Verification items for the finished model (mm, model axes). A direction names the side the tool comes from. Give positions to 0.01 mm unless a question says otherwise; leave off trailing zeros. Loops run counter-clockwise (first coordinate to the right, second up) from the corner with the lowest first, then second, coordinate; pieces in that order, holes last. Notation, with made-up numbers: (85, -19.5) - (94, -19.5) arc R6 cw to (94, -15.5) - close; hole circle Ø10 at (62, -39.75). An arc over 180 degrees is marked (long way). One line per question, with ' | ' between items. Start each with the question number.
1. Section check D-D, the plane y = 85. Enter the section's corners in (x, z).
2. Section check B-B, the plane y = -36. Enter the section's corners in (x, z).
3. Thickness scan on line 1 along Z through (x, y) = (123, -98); line 2 along Z through (x, y) = (151, 86.5); line 3 along Y through (x, z) = (0, 219). Record the ranges inside material, lowest first. Write a range as from..to.
4. Tool access check on faces 4 (the face through (-150, 27, 324)), 5 (the face through (175.35, 91.76, 332.37)), 6 (the face through (-1.08, -4.88, 9.86)). Record the directions out of +Z, -Z, +X, -X, +Y, -Y that give a thin tool (end or side, any length) a straight path to the whole face; none if there is none.
5. Mould release check, pull along Y, two halves, no side actions. Record for faces 1 (the face through (-80, -138, 324)), 2 (the face through (-1.08, -4.88, 219.86)), 3 (the face through (115.962, -111.586, 113.67)): +Y half, -Y half, draft (parallel to the pull), parting line (faces both ways), or undercut.
6. Depth check by flat-ended pin: pin 1 Ø12 at (y, z) = (85, 325) entering from +X; pin 2 Ø11.5 at (x, y) = (0, 0) entering from +Z; pin 3 Ø3 at (x, z) = (103.5, 329.5) entering from -Y; pin 4 Ø5 at (y, z) = (90.5, 97.5) entering from +X. Enter the tip coordinate at first touch or a pass-through.
7. Section check A-A, the plane z = 325. Enter the section's corners in (x, y), then the cut area to 3 significant figures.
8. Section check C-C, the plane z = 182.5. Enter the section's corners in (x, y).
from build123d import *

# Parameters (mm, degrees)
SKETCH1_R           = 5
BOSS_EXTRUDE1_DEPTH = 440
CUT_EXTRUDE2_START  = -420
SKETCH2_R           = 5
CUT_EXTRUDE2_DEPTH  = 420
BOSS_EXTRUDE2_START = -20
SKETCH3_R           = 5
BOSS_EXTRUDE2_DEPTH = 20
BOSS_EXTRUDE3_START = -20
SKETCH4_R           = 5
BOSS_EXTRUDE3_DEPTH = 20
CUT_EXTRUDE3_DEPTH  = 190
CUT_EXTRUDE4_START  = 190
CUT_EXTRUDE4_DEPTH  = 190
SKETCH8_R           = 10
CUT_EXTRUDE5_DEPTH  = 190
BOSS_EXTRUDE4_START = 30
SKETCH9_R           = 12.5
SKETCH9_R_2         = 10
BOSS_EXTRUDE4_DEPTH = 30
BOSS_EXTRUDE5_DEPTH = 440


with BuildPart() as part:
    # Sketch1 → Boss-Extrude1 (new body)
    with BuildSketch(Plane.XY):
        with BuildLine():
            Line((-170, 140), (170, 140))
            Line((170, 140), (170, -100))
            ThreePointArc((170, -100), (0, -160), (-170, -100))
            Line((-170, -100), (-170, 140))
        make_face()
        Circle(SKETCH1_R, mode=Mode.SUBTRACT)
    extrude(amount=BOSS_EXTRUDE1_DEPTH)

    # Sketch2 → Cut-Extrude2 (cut)
    with BuildSketch(Plane.XY.offset(440).offset(CUT_EXTRUDE2_START)):
        with BuildLine():
            Line((150, 140), (-150, 140))
            Line((-150, 140), (-150, -90.207361828))
            ThreePointArc((-150, -90.207361828), (0, -140), (150, -90.207361828))
            Line((150, -90.207361828), (150, 140))
        make_face()
        Circle(SKETCH2_R, mode=Mode.SUBTRACT)
    extrude(amount=CUT_EXTRUDE2_DEPTH, mode=Mode.SUBTRACT)

    # Sketch3 → Boss-Extrude2 (add)
    with BuildSketch(Plane.XY.offset(440).offset(BOSS_EXTRUDE2_START)):
        with BuildLine():
            Line((-150, 140), (-150, -90.207361828))
            ThreePointArc((-150, -90.207361828), (0, -140), (150, -90.207361828))
            Line((150, -90.207361828), (150, 140))
            Line((150, 140), (-150, 140))
        make_face()
        Circle(SKETCH3_R, mode=Mode.SUBTRACT)
    extrude(amount=BOSS_EXTRUDE2_DEPTH)

    # Sketch4 → Boss-Extrude3 (add)
    with BuildSketch(Plane.XY.offset(230).offset(BOSS_EXTRUDE3_START)):
        with BuildLine():
            Line((-170, 140), (-170, -100))
            ThreePointArc((-170, -100), (0, -160), (170, -100))
            Line((170, -100), (170, 140))
            Line((170, 140), (-170, 140))
        make_face()
        Circle(SKETCH4_R, mode=Mode.SUBTRACT)
    extrude(amount=BOSS_EXTRUDE3_DEPTH)

    # Sketch6 → Cut-Extrude3 (cut)
    with BuildSketch(Plane.XY.offset(230)):
        with BuildLine():
            Line((-80, -157.872832651), (-80, -126.403399298))
            ThreePointArc((-80, -126.403399298), (0, -139.528938804), (80, -126.403399298))
            Line((80, -126.403399298), (80, -157.872832651))
            ThreePointArc((80, -157.872832651), (0, -169.528938804), (-80, -157.872832651))
        make_face()
    extrude(amount=CUT_EXTRUDE3_DEPTH, mode=Mode.SUBTRACT)

    # Sketch7 → Cut-Extrude4 (cut)
    with BuildSketch(Plane(origin=(0, 0, 210), x_dir=(-1, 0, 0), z_dir=(0, 0, -1)).offset(CUT_EXTRUDE4_START)):
        with BuildLine():
            Line((-80, -126.900469714), (-80, -160.673360289))
            ThreePointArc((-80, -160.673360289), (0, -172.214162118), (80, -160.673360289))
            Line((80, -160.673360289), (80, -126.900469714))
            ThreePointArc((80, -126.900469714), (0, -140), (-80, -126.900469714))
        make_face()
    extrude(amount=-CUT_EXTRUDE4_DEPTH, mode=Mode.SUBTRACT)

    # Sketch8 → Cut-Extrude5 (cut)
    with BuildSketch(Plane(origin=(170, 0, 0), x_dir=(0, 0, -1), z_dir=(1, 0, 0))):
        with Locations((-325, 85)):
            Circle(SKETCH8_R)
        with Locations((-115, 85)):
            Circle(SKETCH8_R)
    extrude(amount=-CUT_EXTRUDE5_DEPTH, mode=Mode.SUBTRACT)

    # Sketch9 → Boss-Extrude4 (add)
    # profile 1 of 2: a face of its own
    with BuildSketch(Plane(origin=(170, 0, 0), x_dir=(0, 0, -1), z_dir=(1, 0, 0)).offset(BOSS_EXTRUDE4_START)):
        with Locations(Location((-325, 85, 0), (0, 0, 180))):
            Circle(SKETCH9_R)
        with Locations((-325, 85)):
            Circle(SKETCH9_R_2, mode=Mode.SUBTRACT)
    # profile 2 of 2: a face of its own
    with BuildSketch(Plane(origin=(170, 0, 0), x_dir=(0, 0, -1), z_dir=(1, 0, 0)).offset(BOSS_EXTRUDE4_START)):
        with Locations(Location((-115, 85, 0), (0, 0, 180))):
            Circle(SKETCH9_R)
        with Locations((-115, 85)):
            Circle(SKETCH9_R_2, mode=Mode.SUBTRACT)
    extrude(amount=-BOSS_EXTRUDE4_DEPTH)

    # Sketch10 → Boss-Extrude5 (add)
    with BuildSketch(Plane(origin=(0, 0, 0), x_dir=(-1, 0, 0), z_dir=(0, 0, -1))):
        with BuildLine():
            Line((-170, -100), (-170, -107.237017076))
            ThreePointArc((-170, -107.237017076), (0, -165.671056736), (170, -107.237017076))
            Line((170, -107.237017076), (170, -100))
            ThreePointArc((170, -100), (0, -160), (-170, -100))
        make_face()
    extrude(amount=-BOSS_EXTRUDE5_DEPTH)


solid = part.part
Results list:
1) outline: (-170, 0) - (170, 0) - (170, 102.5) - (200, 102.5) - (200, 105) - (150, 105) - (150, 20) - (-150, 20) - (-150, 210) - (150, 210) - (150, 125) - (200, 125) - (200, 127.5) - (170, 127.5) - (170, 312.5) - (200, 312.5) - (200, 315) - (150, 315) - (150, 230) - (-150, 230) - (-150, 420) - (150, 420) - (150, 335) - (200, 335) - (200, 337.5) - (170, 337.5) - (170, 440) - (-170, 440) - close
2) outline: (-170, 0) - (170, 0) - (170, 440) - (-170, 440) - close; hole (-150, 20) - (150, 20) - (150, 210) - (-150, 210) - close; hole (-150, 230) - (150, 230) - (150, 420) - (-150, 420) - close
3) line 1: 0..20, 210..230, 420..440 | line 2: 0..105.11, 124.89..315.11, 334.89..440 | line 3: -165.67..-5, 5..140
4) face 4: +Y | face 5: +X | face 6: +Z, -Z
5) face 1: draft | face 2: undercut | face 3: +Y half
6) pin 1: x = -150 | pin 2: z = 440 | pin 3: y = -146.17 | pin 4: x = 170
7) outline: (-170, -107.24) arc R276.5 ccw to (170, -107.24) - (170, 72.5) - (200, 72.5) - (200, 75) - (150, 75) - (150, -90.21) arc R250.83 cw to (80, -126.9) - (80, -147.91) arc R270.83 cw to (-80, -147.91) - (-80, -126.9) arc R250.83 cw to (-150, -90.21) - (-150, 140) - (-170, 140) - close; (150, 95) - (200, 95) - (200, 97.5) - (170, 97.5) - (170, 140) - (150, 140) - close | area: 14,900 mm²
8) outline: (-170, -107.24) arc R276.5 ccw to (170, -107.24) - (170, 140) - (150, 140) - (150, -90.21) arc R250.83 cw to (80, -126.9) - (80, -147.91) arc R270.83 cw to (-80, -147.91) - (-80, -126.9) arc R250.83 cw to (-150, -90.21) - (-150, 140) - (-170, 140) - close
